Source: three-view drawing plus pictorial views. Frame: mm from the lowest corner of the part. A direction names the side the tool comes from. Give positions to 0.01 mm unless a question says otherwise; leave off trailing zeros. Loops run counter-clockwise (first coordinate to the right, second up) from the corner with the lowest first, then second, coordinate; pieces in that order, holes last. Notation, with made-up numbers: M 68,89.5 L 81,89.5 A27 ccw 81,105.5 Z; hole C 72.25,-38.75 d9. An arc over 180 degrees is marked long. Answer as a JSON object with one key per item and string values. Group by question number.
1) Access query for the marked faces 1 and 2. Directions: +Z, -Z, +X, -X, +Y, -Y. A direction counts if a zero-diameter tool reaches every point of the face in a straight line with its end or side. Return the directions, or none.
2) Ray query, L1, parallel to Y at x = 7.75, z = 5.5. Return the intervals inside material, ascending.
3) Section query C-C on x = 1. Return loops of the section in (y, z).
4) Section query A-A on z = 5. Return loops of the section in (x, y), plus the area to 3 significant figures.
5) Section query B-B on x = 4.75. Return loops of the section in (y, z) (1 decimal).
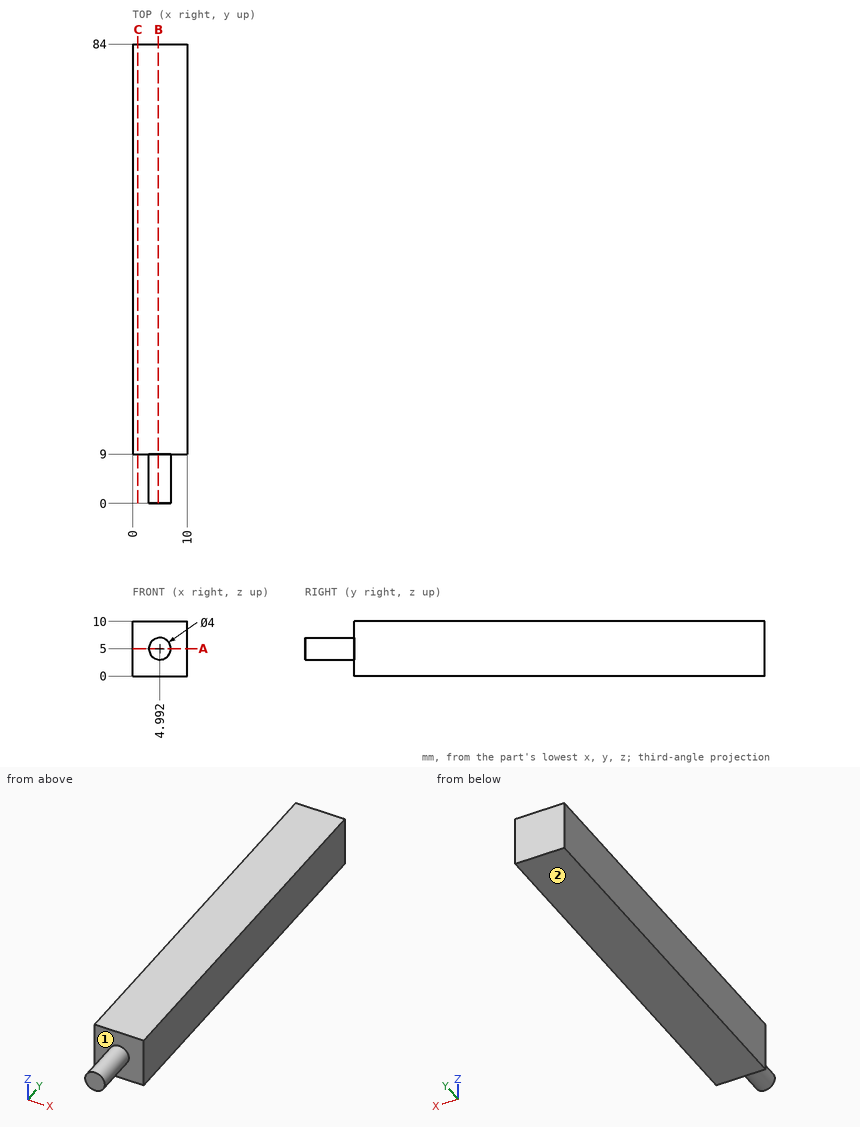
Output:
{
 "1": {"face 1": "-Y", "face 2": "-Z, +X, -X, +Y, -Y"},
 "2": {"L1": "y = 9 to 84"},
 "3": {"outline": "M 9,0 L 84,0 L 84,10 L 9,10 Z"},
 "4": {"outline": "M 0,9 L 2.99,9 L 2.99,0 L 6.99,0 L 6.99,9 L 10,9 L 10,84 L 0,84 Z", "area": "786 mm^2"},
 "5": {"outline": "M 0,3 L 9,3 L 9,0 L 84,0 L 84,10 L 9,10 L 9,7 L 0,7 Z"}
}
